Work out the finished part from the listing and answer in its coordinate system (mm). A direction names the side the tool comes from. Round coordinates to 2 decimals unless told otherwise and drop trailing zeros. Write each loop counter-clockwise with the first axis right and the second up, starting at its lowest first coordinate (ties: lowest second). Pieces come first, ordered by that corner, then holes.
1. A tool of negligible diameter and unlimited length cuts with its end or side. For faces 1 (the face through (24, 0, -3)), 2 (the face through (-18.89, 0.51, 174.15)), from which of +Z, -Z, +X, -X, +Y, -Y can it reach the whole face along a straight path? Write none if from no direction.
2. Find section A-A (z = 142.5). Write down the section's boundary in (x, y).
3. Straight lines are drawn through the part: probe 1 along X at (y, z) = (0.7, 215); probe 2 along X at (y, z) = (0.85, -146.5); probe 3 along Z at (x, y) = (49, 0.9). For each, find the intervals that lie inside material, in ascending order.
4. Determine the mould class of faces 3 (the face through (24, 1, -3)), 4 (the face through (18.89, 0.51, 174.15)) for opening direction X: pulls with the +X half, pulls with the -X half, needs draft (parallel to the pull), parting line crosses it, or undercut.
5. Flat-ended cylindrical pins translate along their axes: pin 1 Ø0.5 at (x, y) = (33.5, 0.5) entering from +Z; pin 2 Ø5 at (x, z) = (47.4, 215) entering from -Y; pin 3 Ø0.5 at (y, z) = (0.5, -231) entering from +X; pin 4 Ø0.5 at (y, z) = (0.5, -222.5) entering from +X. Find the tip coordinate at first contact, or state that the pin passes through.
6. Find section B-B (y = 0.35). Count the separate pieces of the cut face and the enclosed holes in it, and give its area (3 significant figures).
```python
from build123d import *

# Parameters (mm, degrees)
SKETCH1_R           = 2.15
SKETCH1_W           = 43.8
SKETCH1_H           = 354
BOSS_EXTRUDE1_DEPTH = 1
FILLET2_R           = 10


with BuildPart() as part:
    # Sketch1 → Boss-Extrude1 (new body)
    with BuildSketch(Plane(origin=(0, 0, 0), x_dir=(1, 0, 0), z_dir=(0, 1, 0))):
        Polygon((-54.9, -221), (-36.9, -221), (-36.9, -225), (-31.9, -225), (-31.9, -241), (31.9, -241), (31.9, -225), (36.9, -225), (36.9, -221), (54.9, -221), (54.9, 221), (36.9, 221), (36.9, 225), (31.9, 225), (31.9, 241), (-31.9, 241), (-31.9, 225), (-36.9, 225), (-36.9, 221), (-54.9, 221), align=None)
        with Locations(Location((-47.4, 175, 0), (0, 0, 270))):
            Circle(SKETCH1_R, mode=Mode.SUBTRACT)
        with Locations(Location((47.4, 175, 0), (0, 0, 270))):
            Circle(SKETCH1_R, mode=Mode.SUBTRACT)
        with Locations(Location((-47.4, -175, 0), (0, 0, 270))):
            Circle(SKETCH1_R, mode=Mode.SUBTRACT)
        with Locations(Location((47.4, -175, 0), (0, 0, 270))):
            Circle(SKETCH1_R, mode=Mode.SUBTRACT)
        with Locations(Location((-47.4, -215, 0), (0, 0, 270))):
            Circle(SKETCH1_R, mode=Mode.SUBTRACT)
        with Locations(Location((47.4, -215, 0), (0, 0, 270))):
            Circle(SKETCH1_R, mode=Mode.SUBTRACT)
        with Locations(Location((47.4, 215, 0), (0, 0, 270))):
            Circle(SKETCH1_R, mode=Mode.SUBTRACT)
        with Locations(Location((-47.4, 215, 0), (0, 0, 270))):
            Circle(SKETCH1_R, mode=Mode.SUBTRACT)
        with Locations(Location((0, 236, 0), (0, 0, 270))):
            Circle(SKETCH1_R, mode=Mode.SUBTRACT)
        with Locations(Location((0, -236, 0), (0, 0, 270))):
            Circle(SKETCH1_R, mode=Mode.SUBTRACT)
        Rectangle(SKETCH1_W, SKETCH1_H, mode=Mode.SUBTRACT)
    extrude(amount=BOSS_EXTRUDE1_DEPTH)

    # Fillet2
    fillet2_edges = [part.edges().sort_by_distance(p)[0] for p in [
        (21.9, 0.5, 177),
        (21.9, 0.5, -177),
        (-21.9, 0.5, -177),
        (-21.9, 0.5, 177),
    ]]
    fillet(fillet2_edges, radius=FILLET2_R)


solid = part.part
```
Worked answers:
1. face 1: +Z, -Z, +X, -X, -Y
1. face 2: +Y, -Y
2. outline: (-54.9, 0) - (-21.9, 0) - (-21.9, 1) - (-54.9, 1) - close; (21.9, 0) - (54.9, 0) - (54.9, 1) - (21.9, 1) - close
3. probe 1: x = -54.9 to -49.55, -45.25 to 45.25, 49.55 to 54.9
3. probe 2: x = -54.9 to -21.9, 21.9 to 54.9
3. probe 3: z = -221 to -216.44, -213.56 to -176.44, -173.56 to 173.56, 176.44 to 213.56, 216.44 to 221
4. face 3: needs draft
4. face 4: undercut
5. pin 1: stops at z = 225
5. pin 2: stops at y = 0
5. pin 3: stops at x = 31.9
5. pin 4: stops at x = 36.9
6. separate pieces: 1
6. enclosed holes: 11
6. area: 35,600 mm2
